Geometry check sheet. Reference: the model listing, model coordinates, mm. A direction names the side the tool comes from. Give positions to 0.01 mm unless a question says otherwise; leave off trailing zeros. Write each loop counter-clockwise with the first axis right and the second up, starting at its lowest first coordinate (ties: lowest second). Pieces come first, ordered by that corner, then holes. Notation, with made-up numbers: M 75,30.5 L 127,30.5 A19 cw 127,39.5 Z; hole C -11,25 d6. An arc over 180 degrees is marked long. One line per item, written item: value. Start each with the question number.
1. Gauge pin test, flat ends, axial feed: pin 1 (5 mm diameter, centred on x = 6.5, z = 42.5, fed in from -Y); pin 2 (10 mm diameter, centred on y = 55.5, z = 23.5, fed in from +X) (3 decimals); pin 3 (1.5 mm diameter, centred on x = 19, y = 64, fed in from -Z); pin 4 (5 mm diameter, centred on y = 118, z = 43, fed in from -X). Record the tip position at first contact, or that the pin passes through.
2. Tool access check on faces 1 (the face through (0, 128, 61)), 2 (the face through (-3.13, 74.93, 31.41)), 3 (the face through (31.706, 119.954, 57.635)), 4 (the face through (31.71, 74.93, 31.41)), 5 (the face through (1.588, 70, 28)). Record the directions out of +Z, -Z, +X, -X, +Y, -Y that give a thin tool (end or side, any length) a straight path to the whole face; none if there is none.
3. Cross-section at D-D on x = 21. Record the cut outline in (y, z).
4. Scan lines: line 1 (X direction, y = 73.5, z = 23.5) (3 decimals); line 2 (Y direction, x = 19, z = 57); line 3 (Z direction, x = 20, y = 109.5). Record each from-to range of solid material in increasing order.
5. Cross-section at B-B on z = 22.5. Record the cut outline in (x, y) (1 decimal), then the cut area to 3 significant figures.
6. Cross-section at A-A on x = 31.5. Record the cut outline in (y, z).
7. Cross-section at C-C on y = 47. Record the cut outline in (x, z) (1 decimal).
from build123d import *

# Parameters (mm, degrees)
BOSS_EXTRUDE1_DEPTH   = 28.575
SKETCH2_W             = 25.4
SKETCH2_H             = 14.2875
CUT_EXTRUDE2_DEPTH    = 159.114345309
CUT_EXTRUDE3_DEPTH    = 29.575
CUT_EXTRUDE4_DEPTH    = 25.4
SKETCH6_W             = 1.5875
SKETCH6_H             = 82.55
BOSS_EXTRUDE2_DEPTH   = 1.5875
CUT_EXTRUDE5_DEPTH    = 29.575
CUT_EXTRUDE6_DEPTH    = 29.575
BOSS_EXTRUDE3_DEPTH   = 6.35
BOSS_EXTRUDE3_2_DEPTH = 6.35
BOSS_EXTRUDE3_3_DEPTH = 6.35


with BuildPart() as part:
    # Sketch1 → Boss-Extrude1 (new body)
    with BuildSketch(Plane(origin=(0, 0, 0), x_dir=(0, 0, -1), z_dir=(1, 0, 0))):
        Polygon((0, 0), (-76.2, 131.982271537), (-59.79061761, 137.95479829), (16.40938239, 5.972526753), align=None)
    extrude(amount=BOSS_EXTRUDE1_DEPTH)

    # Sketch2 → Cut-Extrude2 (cut, through all, along a direction that is not the sketch's normal)
    with BuildSketch(Plane(origin=(0, 141.033486548, 51.331991138), x_dir=(1, 0, 0), z_dir=(0, 0.939692621, 0.342020143))):
        with Locations((14.2875, -17.732732276)):
            Rectangle(SKETCH2_W, SKETCH2_H)
    extrude(amount=-CUT_EXTRUDE2_DEPTH, dir=(0, 0.866025404, 0.5), mode=Mode.SUBTRACT)

    # Sketch3 → Cut-Extrude3 (cut, through all)
    with BuildSketch(Plane(origin=(28.575, 0, 0), x_dir=(0, 0, -1), z_dir=(1, 0, 0))):
        Polygon((-76.2, 131.982271537), (-74.708237965, 132.525228514), (-33.433237965, 61.034831432), (-34.925, 60.491874454), align=None)
    extrude(amount=-CUT_EXTRUDE3_DEPTH, mode=Mode.SUBTRACT)

    # Sketch4 → Cut-Extrude4 (cut)
    with BuildSketch(Plane(origin=(1.5875, 0, 0), x_dir=(0, 0, -1), z_dir=(1, 0, 0))):
        Polygon((-43.162002392, 69.198234075), (-23.704473537, 52.871428789), (-24.724898867, 51.655333235), (-44.182427722, 67.982138521), align=None)
    extrude(amount=CUT_EXTRUDE4_DEPTH, mode=Mode.SUBTRACT)

    # Sketch6 → Boss-Extrude2 (add, along a direction that is not the sketch's normal)
    with BuildSketch(Plane(origin=(0, 0.781691154, -1.353928794), x_dir=(1, 0, 0), z_dir=(0, -0.5, 0.866025404))):
        with Locations((27.78125, 110.849333518)):
            Rectangle(SKETCH6_W, SKETCH6_H)
        with Locations((0.79375, 110.849333518)):
            Rectangle(SKETCH6_W, SKETCH6_H)
    extrude(amount=BOSS_EXTRUDE2_DEPTH, dir=(0, -0.342020143, 0.939692621))

    # Sketch7 → Cut-Extrude5 (cut, through all)
    with BuildSketch(Plane(origin=(28.575, 0, 0), x_dir=(0, 0, -1), z_dir=(1, 0, 0))):
        Polygon((-76.2, 131.982271537), (-71.724713894, 133.611142469), (-63.568463887, 119.484103058), (-68.043749993, 117.855232125), align=None)
    extrude(amount=-CUT_EXTRUDE5_DEPTH, mode=Mode.SUBTRACT)

    # Sketch8 → Cut-Extrude6 (cut, through all)
    with BuildSketch(Plane(origin=(28.575, 0, 0), x_dir=(0, 0, -1), z_dir=(1, 0, 0))):
        Polygon((-68.043749993, 117.855232125), (-65.060225922, 118.94114608), (2.983524071, 1.085913955), (0, 0), align=None)
    extrude(amount=-CUT_EXTRUDE6_DEPTH, mode=Mode.SUBTRACT)


with BuildPart() as body_2:
    # Sketch9 → Boss-Extrude3 (new body)
    with BuildSketch(Plane(origin=(28.575, 0, 0), x_dir=(0, 0, -1), z_dir=(1, 0, 0))):
        Polygon((-64.254231049, 117.545122009), (-50.828372729, 122.431734807), (-47.653372729, 116.932473493), (-61.079231049, 112.045860695), align=None)
    extrude(amount=BOSS_EXTRUDE3_DEPTH)


with BuildPart() as body_3:
    # Sketch9 → Boss-Extrude3 2 (new body)
    with BuildSketch(Plane(origin=(28.575, 0, 0), x_dir=(0, 0, -1), z_dir=(1, 0, 0))):
        Polygon((-41.394231049, 77.950440548), (-27.968372729, 82.837053346), (-24.793372729, 77.337792032), (-38.219231049, 72.451179234), align=None)
    extrude(amount=BOSS_EXTRUDE3_2_DEPTH)


with BuildPart() as body_4:
    # Sketch9 → Boss-Extrude3 3 (new body)
    with BuildSketch(Plane(origin=(28.575, 0, 0), x_dir=(0, 0, -1), z_dir=(1, 0, 0))):
        Polygon((-18.534231049, 38.355759087), (-5.108372729, 43.242371885), (-1.933372729, 37.743110571), (-15.359231049, 32.856497773), align=None)
    extrude(amount=BOSS_EXTRUDE3_3_DEPTH)


with BuildPart() as body_5:
    # Mirror1: mirrored copy
    add(body_2.part.mirror(Plane.ZY.offset(-14.2875)))


with BuildPart() as body_6:
    # Mirror1 2: mirrored copy
    add(body_3.part.mirror(Plane.ZY.offset(-14.2875)))


with BuildPart() as body_7:
    # Mirror1 3: mirrored copy
    add(body_4.part.mirror(Plane.ZY.offset(-14.2875)))


with BuildPart() as part_1:
    add(part.part)

    # Combine1: union body 2, body 3, body 4, body 7, body 6, body 5
    add(body_2.part)
    add(body_3.part)
    add(body_4.part)
    add(body_7.part)
    add(body_6.part)
    add(body_5.part)


solid = part_1.part
Report:
1. pin 1: stops at y = 100.55
1. pin 2: stops at x = 28.575
1. pin 3: stops at z = 16.66
1. pin 4: passes through
2. face 1: +Z, -X, +Y
2. face 2: -Z, -X, -Y
2. face 3: +Z, +X, +Y
2. face 4: -Z, +X, -Y
2. face 5: +Z, -Y
3. outline: M 5.43,-14.92 L 5.97,-16.41 L 137.95,59.79 L 137.41,61.28 Z
4. line 1: x = 0 to 28.575
4. line 2: y = 129.99 to 133.12
4. line 3: z = 43.36 to 45.17
5. outline: M 0,45.2 L 1.6,45.2 L 1.6,70.2 L 27,70.2 L 27,45.2 L 28.6,45.2 L 28.6,73.4 L 0,73.4 Z
5. area: 169 mm^2
6. outline: M 32.86,15.36 L 37.74,1.93 L 43.24,5.11 L 38.36,18.53 Z; M 72.45,38.22 L 77.34,24.79 L 82.84,27.97 L 77.95,41.39 Z; M 112.05,61.08 L 116.93,47.65 L 122.43,50.83 L 117.55,64.25 Z
7. outline: M 0,7.3 L 28.6,7.3 L 28.6,23.5 L 27,23.5 L 27,9.1 L 1.6,9.1 L 1.6,23.5 L 0,23.5 Z
